Geometry check sheet. Reference: the model listing, model coordinates, mm. A direction names the side the tool comes from. Give positions to 0.01 mm unless a question says otherwise; leave off trailing zeros. Order: outer loops, then holes, each group sorted by start corner. A loop starts at its lowest first (then second) coordinate and runs counter-clockwise, first axis right, second up. Notation, with made-up numbers: M -9,-25 L -3,-25 A22 ccw -3,5 Z; hole C 75.5,54.25 d8. An arc over 180 degrees is marked long. Answer as CSV lines item,"result". Start each with the question number.
Q1. Go/stop test with flat-tipped pins: pin 1 (4 mm diameter, centred on x = -18.61, z = 6, fed in from -Y); pin 2 (5.5 mm diameter, centred on x = 21.5, z = 6, fed in from +Y); pin 3 (5.5 mm diameter, centred on x = 19.5, z = 7, fed in from +Y); pin 4 (4 mm diameter, centred on x = 8, z = 2.5, fed in from -Y). Record where each tip stops, or that it passes through.
Q2. Thickness scan on line 1 (X direction, y = -3.5, z = 0.75); line 2 (X direction, y = -9, z = 4); line 3 (X direction, y = 8, z = 2). Record the ranges inside material, lowest first.
Q3. Set-up check for faces 4 (the flat face through (-15.5, -2, 6)), 5 (the flat face through (16.29, -7, 6)), 6 (the flat face through (15.364, -3, 6)), 7 (the flat face through (12.5, -6, 6)): record each of +Z, -Z, +X, -X, +Y, -Y from which the full face is reachable in a straight line by a thin tool's end or side.
Q4. Mould release check, pull along X, two halves, no side actions. Record for faces 1 (the flat face through (20.206, -7.779, 3.76)), 2 (the cylindrical face through (1.38, 15.44, 5.92)), 3 (the flat face through (22, -6.3, 6)): +X half, -X half, draft (parallel to the pull), parting line (faces both ways), or undercut.
Q5. Section check A-A, the plane z = 6. Count the separate pieces of the cut face and the enclosed holes in it, then the cut area to 3 significant figures.
Q6. Section check D-D, the plane x = 0. Record the boundary of the cut face in (y, z).
Q7. Section check B-B, the plane y = 4.25. Record the boundary of the cut face in (x, z), then the cut area to 3 significant figures.
Q8. Section check C-C, the plane z = 1. Record the boundary of the cut face in (x, y), then the cut area to 3 significant figures.
```python
from build123d import *

# Parameters (mm, degrees)
BOSS_EXTRUDE1_DEPTH = 12
SKETCH2_R           = 1.65
CUT_EXTRUDE1_DEPTH  = 35.49487292
CUT_EXTRUDE2_DEPTH  = 3
FILLET2_R           = 3
FILLET3_R           = 0.3


with BuildPart() as part:
    # Sketch1 → Boss-Extrude1 (new body)
    with BuildSketch(Plane.XY):
        with BuildLine():
            Line((-12.5, -12.5), (-12.5, 0))
            ThreePointArc((-12.5, 0), (0, 12.5), (12.5, 0))
            Line((12.5, 0), (12.5, -12.5))
            Line((12.5, -12.5), (23.888412626, -12.5))
            Line((23.888412626, -12.5), (23.888412626, -6.3))
            Line((23.888412626, -6.3), (15.363999686, -6.3))
            Line((15.363999686, -6.3), (15.363999686, -2.048783456))
            ThreePointArc((15.363999686, -2.048783456), (1.026646207, 15.465962549), (-15.5, 0))
            Line((-15.5, 0), (-15.5, -6.3))
            Line((-15.5, -6.3), (-23.612861565, -6.3))
            Line((-23.612861565, -6.3), (-23.612861565, -12.5))
            Line((-23.612861565, -12.5), (-12.5, -12.5))
        make_face()
    extrude(amount=BOSS_EXTRUDE1_DEPTH)

    # Sketch2 → Cut-Extrude1 (cut, through all)
    with BuildSketch(Plane(origin=(0, -6.3, 0), x_dir=(1, 0, 0), z_dir=(0, 1, 0))):
        with Locations(Location((-18.612861565, -6, 0), (0, 0, 180))):
            Circle(SKETCH2_R)
        with Locations(Location((18.888412626, -6, 0), (0, 0, 180))):
            Circle(SKETCH2_R)
    extrude(amount=-CUT_EXTRUDE1_DEPTH, mode=Mode.SUBTRACT)

    # Sketch3 → Cut-Extrude2 (cut)
    with BuildSketch(Plane(origin=(0, -6.3, 0), x_dir=(1, 0, 0), z_dir=(0, 1, 0))):
        Polygon((18.888412626, -3), (16.290336415, -4.5), (16.290336415, -7.5), (18.888412626, -9), (21.486488837, -7.5), (21.486488837, -4.5), align=None)
        Polygon((-18.612861565, -9), (-16.014785354, -7.5), (-16.014785354, -4.5), (-18.612861565, -3), (-21.210937777, -4.5), (-21.210937777, -7.5), align=None)
    extrude(amount=-CUT_EXTRUDE2_DEPTH, mode=Mode.SUBTRACT)

    # Fillet2
    # the kernel refuses this fillet: 3 mm, written as the material it adds along each edge
    with BuildSketch(Plane(origin=(-15.5, -6.3, 0), x_dir=(0, 1, 0), z_dir=(0, 0, 1))) as fillet2_piece_1_section:
        with BuildLine():
            CenterArc((FILLET2_R, FILLET2_R), FILLET2_R, 180, 90)
            Line((0, FILLET2_R), (0, 0))
            Line((0, 0), (FILLET2_R, 0))
        make_face()
    fillet2_piece_1 = extrude(amount=12, mode=Mode.PRIVATE)
    fillet2_piece_1 = split(fillet2_piece_1, bisect_by=Plane(origin=(-16.699597169, -5.271939642, 4.104623714), z_dir=(0.5000000000000008, 0, -0.8660254037844383)), keep=Keep.TOP, mode=Mode.PRIVATE)
    fillet2_piece_1 = split(fillet2_piece_1, bisect_by=Plane(origin=(-16.014785354, -5.271939642, 2.345499265), z_dir=(1, 0, 0)), keep=Keep.TOP, mode=Mode.PRIVATE)
    add(fillet2_piece_1)
    with BuildSketch(Plane(origin=(-15.5, -6.3, 0), x_dir=(0, 1, 0), z_dir=(0, 0, 1))) as fillet2_piece_2_section:
        with BuildLine():
            CenterArc((FILLET2_R, FILLET2_R), FILLET2_R, 180, 90)
            Line((0, FILLET2_R), (0, 0))
            Line((0, 0), (FILLET2_R, 0))
        make_face()
    fillet2_piece_2 = extrude(amount=12, mode=Mode.PRIVATE)
    fillet2_piece_2 = split(fillet2_piece_2, bisect_by=Plane(origin=(-17.543441621, -5.964994309, 3.617429893), z_dir=(0.5000000000000008, 0, -0.8660254037844383)), keep=Keep.TOP, mode=Mode.PRIVATE)
    fillet2_piece_2 = split(fillet2_piece_2, bisect_by=Plane(origin=(-16.014785354, -5.964994309, 2.067102796), z_dir=(-1, 0, 0)), keep=Keep.TOP, mode=Mode.PRIVATE)
    add(fillet2_piece_2)
    with BuildSketch(Plane(origin=(-15.5, -6.3, 0), x_dir=(0, 1, 0), z_dir=(0, 0, 1))) as fillet2_piece_3_section:
        with BuildLine():
            CenterArc((FILLET2_R, FILLET2_R), FILLET2_R, 180, 90)
            Line((0, FILLET2_R), (0, 0))
            Line((0, 0), (FILLET2_R, 0))
        make_face()
    fillet2_piece_3 = extrude(amount=12, mode=Mode.PRIVATE)
    fillet2_piece_3 = split(fillet2_piece_3, bisect_by=Plane(origin=(-15.128726527, -5.296162819, 5.011566302), z_dir=(-0.5000000000000008, 0, 0.8660254037844383)), keep=Keep.TOP, mode=Mode.PRIVATE)
    fillet2_piece_3 = split(fillet2_piece_3, bisect_by=Plane(origin=(-16.014785354, -5.296162819, 6), z_dir=(1, 0, 0)), keep=Keep.TOP, mode=Mode.PRIVATE)
    fillet2_piece_3 = split(fillet2_piece_3, bisect_by=Plane(origin=(-15.128726527, -5.296162819, 6.988433698), z_dir=(-0.49999999999999994, 0, -0.8660254037844389)), keep=Keep.TOP, mode=Mode.PRIVATE)
    add(fillet2_piece_3)
    with BuildSketch(Plane(origin=(-15.5, -6.3, 0), x_dir=(0, 1, 0), z_dir=(0, 0, 1))) as fillet2_piece_4_section:
        with BuildLine():
            CenterArc((FILLET2_R, FILLET2_R), FILLET2_R, 180, 90)
            Line((0, FILLET2_R), (0, 0))
            Line((0, 0), (FILLET2_R, 0))
        make_face()
    fillet2_piece_4 = extrude(amount=12, mode=Mode.PRIVATE)
    fillet2_piece_4 = split(fillet2_piece_4, bisect_by=Plane(origin=(-16.014785354, -5.271939642, 9.654500735), z_dir=(1, 0, 0)), keep=Keep.TOP, mode=Mode.PRIVATE)
    fillet2_piece_4 = split(fillet2_piece_4, bisect_by=Plane(origin=(-16.699597169, -5.271939642, 7.895376286), z_dir=(0.49999999999999994, 0, 0.8660254037844389)), keep=Keep.TOP, mode=Mode.PRIVATE)
    add(fillet2_piece_4)
    with BuildSketch(Plane(origin=(-15.5, -6.3, 0), x_dir=(0, 1, 0), z_dir=(0, 0, 1))) as fillet2_piece_5_section:
        with BuildLine():
            CenterArc((FILLET2_R, FILLET2_R), FILLET2_R, 180, 90)
            Line((0, FILLET2_R), (0, 0))
            Line((0, 0), (FILLET2_R, 0))
        make_face()
    fillet2_piece_5 = extrude(amount=12, mode=Mode.PRIVATE)
    fillet2_piece_5 = split(fillet2_piece_5, bisect_by=Plane(origin=(-16.014785354, -5.964994309, 9.932897204), z_dir=(-1, 0, 0)), keep=Keep.TOP, mode=Mode.PRIVATE)
    fillet2_piece_5 = split(fillet2_piece_5, bisect_by=Plane(origin=(-17.543441621, -5.964994309, 8.382570107), z_dir=(0.49999999999999994, 0, 0.8660254037844389)), keep=Keep.TOP, mode=Mode.PRIVATE)
    add(fillet2_piece_5)
    with BuildSketch(Plane(origin=(15.363999686, -6.3, 0), x_dir=(0, 1, 0), z_dir=(0, 0, 1))) as fillet2_piece_6_section:
        with BuildLine():
            CenterArc((FILLET2_R, -FILLET2_R), FILLET2_R, 90, 90)
            Line((0, -FILLET2_R), (0, 0))
            Line((0, 0), (FILLET2_R, 0))
        make_face()
    fillet2_piece_6 = extrude(amount=12, mode=Mode.PRIVATE)
    fillet2_piece_6 = split(fillet2_piece_6, bisect_by=Plane(origin=(16.290336415, -5.412045629, 2.423810939), z_dir=(-1, 0, 0)), keep=Keep.TOP, mode=Mode.PRIVATE)
    fillet2_piece_6 = split(fillet2_piece_6, bisect_by=Plane(origin=(16.737778584, -5.412045629, 4.241669143), z_dir=(-0.4999999999999997, 0, -0.866025403784439)), keep=Keep.TOP, mode=Mode.PRIVATE)
    add(fillet2_piece_6)
    with BuildSketch(Plane(origin=(15.363999686, -6.3, 0), x_dir=(0, 1, 0), z_dir=(0, 0, 1))) as fillet2_piece_7_section:
        with BuildLine():
            CenterArc((FILLET2_R, -FILLET2_R), FILLET2_R, 90, 90)
            Line((0, -FILLET2_R), (0, 0))
            Line((0, 0), (FILLET2_R, 0))
        make_face()
    fillet2_piece_7 = extrude(amount=12, mode=Mode.PRIVATE)
    fillet2_piece_7 = split(fillet2_piece_7, bisect_by=Plane(origin=(16.290336415, -6.100859955, 2.085482464), z_dir=(1, 0, 0)), keep=Keep.TOP, mode=Mode.PRIVATE)
    fillet2_piece_7 = split(fillet2_piece_7, bisect_by=Plane(origin=(17.763282274, -6.100859955, 3.649594312), z_dir=(-0.4999999999999997, 0, -0.866025403784439)), keep=Keep.TOP, mode=Mode.PRIVATE)
    add(fillet2_piece_7)
    with BuildSketch(Plane(origin=(15.363999686, -6.3, 0), x_dir=(0, 1, 0), z_dir=(0, 0, 1))) as fillet2_piece_8_section:
        with BuildLine():
            CenterArc((FILLET2_R, -FILLET2_R), FILLET2_R, 90, 90)
            Line((0, -FILLET2_R), (0, 0))
            Line((0, 0), (FILLET2_R, 0))
        make_face()
    fillet2_piece_8 = extrude(amount=12, mode=Mode.PRIVATE)
    fillet2_piece_8 = split(fillet2_piece_8, bisect_by=Plane(origin=(15.225397876, -5.465952717, 6.885157448), z_dir=(0.5000000000000012, 0, -0.866025403784438)), keep=Keep.TOP, mode=Mode.PRIVATE)
    fillet2_piece_8 = split(fillet2_piece_8, bisect_by=Plane(origin=(16.290336415, -5.465952717, 6), z_dir=(-1, 0, 0)), keep=Keep.TOP, mode=Mode.PRIVATE)
    fillet2_piece_8 = split(fillet2_piece_8, bisect_by=Plane(origin=(15.225397876, -5.465952717, 5.114842552), z_dir=(0.4999999999999997, 0, 0.866025403784439)), keep=Keep.TOP, mode=Mode.PRIVATE)
    add(fillet2_piece_8)
    with BuildSketch(Plane(origin=(15.363999686, -6.3, 0), x_dir=(0, 1, 0), z_dir=(0, 0, 1))) as fillet2_piece_9_section:
        with BuildLine():
            CenterArc((FILLET2_R, -FILLET2_R), FILLET2_R, 90, 90)
            Line((0, -FILLET2_R), (0, 0))
            Line((0, 0), (FILLET2_R, 0))
        make_face()
    fillet2_piece_9 = extrude(amount=12, mode=Mode.PRIVATE)
    fillet2_piece_9 = split(fillet2_piece_9, bisect_by=Plane(origin=(16.737778584, -5.412045629, 7.758330857), z_dir=(-0.5000000000000012, 0, 0.866025403784438)), keep=Keep.TOP, mode=Mode.PRIVATE)
    fillet2_piece_9 = split(fillet2_piece_9, bisect_by=Plane(origin=(16.290336415, -5.412045629, 9.576189061), z_dir=(-1, 0, 0)), keep=Keep.TOP, mode=Mode.PRIVATE)
    add(fillet2_piece_9)
    with BuildSketch(Plane(origin=(15.363999686, -6.3, 0), x_dir=(0, 1, 0), z_dir=(0, 0, 1))) as fillet2_piece_10_section:
        with BuildLine():
            CenterArc((FILLET2_R, -FILLET2_R), FILLET2_R, 90, 90)
            Line((0, -FILLET2_R), (0, 0))
            Line((0, 0), (FILLET2_R, 0))
        make_face()
    fillet2_piece_10 = extrude(amount=12, mode=Mode.PRIVATE)
    fillet2_piece_10 = split(fillet2_piece_10, bisect_by=Plane(origin=(17.763282274, -6.100859955, 8.350405688), z_dir=(-0.5000000000000012, 0, 0.866025403784438)), keep=Keep.TOP, mode=Mode.PRIVATE)
    fillet2_piece_10 = split(fillet2_piece_10, bisect_by=Plane(origin=(16.290336415, -6.100859955, 9.914517536), z_dir=(1, 0, 0)), keep=Keep.TOP, mode=Mode.PRIVATE)
    add(fillet2_piece_10)

    # Fillet3
    fillet3_edges = [part.edges().sort_by_distance(p)[0] for p in [
        (23.888412626, -6.3, 6),
        (23.888412626, -12.5, 6),
        (12.5, -12.5, 6),
        (-12.5, -12.5, 6),
        (-23.612861565, -12.5, 6),
        (-23.612861565, -6.3, 6),
    ]]
    fillet(fillet3_edges, radius=FILLET3_R)


solid = part.part
```
Answer block:
1,pin 1,"stops at y = -12.5"
1,pin 2,"stops at y = -6.3"
1,pin 3,"stops at y = -5.91"
1,pin 4,"stops at y = 7.5"
2,line 1,"x = -15.51 to -12.5, 12.5 to 15.37"
2,line 2,"x = -23.61 to -20.34, -16.88 to -12.5, 12.5 to 17.16, 20.62 to 23.89"
2,line 3,"x = -13.28 to -9.6, 9.6 to 13.28"
3,face 4,"+Z, -Z, -X, +Y"
3,face 5,"+Y"
3,face 6,"+Z, -Z, +X"
3,face 7,"+Z, -Z, -Y"
4,face 1,"undercut"
4,face 2,"parting line"
4,face 3,"draft"
5,separate pieces,"3"
5,enclosed holes,"0"
5,area,"259 mm2"
6,outline,"M 12.5,0 L 15.5,0 L 15.5,12 L 12.5,12 Z"
7,outline,"M -14.91,0 L -11.76,0 L -11.76,12 L -14.91,12 Z; M 11.76,0 L 14.91,0 L 14.91,12 L 11.76,12 Z"
7,area,"75.6 mm2"
8,outline,"M -23.61,-12.2 A0.3 ccw -23.31,-12.5 L -12.8,-12.5 A0.3 ccw -12.5,-12.2 L -12.5,0 A12.5 cw 12.5,0 L 12.5,-12.2 A0.3 ccw 12.8,-12.5 L 23.59,-12.5 A0.3 ccw 23.89,-12.2 L 23.89,-6.6 A0.3 ccw 23.59,-6.3 L 18.36,-6.3 A3 cw 15.36,-3.3 L 15.36,-2.05 A15.5 ccw long -15.5,0 L -15.5,-3.3 A3 cw -18.5,-6.3 L -23.31,-6.3 A0.3 ccw -23.61,-6.6 Z"
8,area,"312 mm2"
